from build123d import *

# Parameters (mm, degrees)
SKETCH_1_R          = 17.5
EXTRUDE_1_DEPTH     = 3.65
SKETCH_3_R          = 1.25
CUT_EXTRUDE_1_DEPTH = 5
CHAMFER_1_SIZE      = 0.5
SKETCH_4_R          = 1.5
CUT_EXTRUDE_2_DEPTH = 10
SKETCH_5_R          = 2.75
CUT_EXTRUDE_3_DEPTH = 10


with BuildPart() as part:
    # 草图1 → 凸台-拉伸1 (new body)
    with BuildSketch(Plane.XY):
        Circle(SKETCH_1_R)
    extrude(amount=EXTRUDE_1_DEPTH)

    # 草图3 → 切除-拉伸1 (cut)
    with BuildSketch(Plane(origin=(0, 0, 0), x_dir=(-1, 0, 0), z_dir=(0, 0, -1))):
        with Locations((0, 13.5)):
            Circle(SKETCH_3_R)
        with Locations((9.545941546, 9.545941546)):
            Circle(SKETCH_3_R)
        with Locations((13.5, 0)):
            Circle(SKETCH_3_R)
        with Locations((9.545941546, -9.545941546)):
            Circle(SKETCH_3_R)
        with Locations((0, -13.5)):
            Circle(SKETCH_3_R)
        with Locations((-9.545941546, -9.545941546)):
            Circle(SKETCH_3_R)
        with Locations((-13.5, 0)):
            Circle(SKETCH_3_R)
        with Locations((-9.545941546, 9.545941546)):
            Circle(SKETCH_3_R)
    extrude(amount=-CUT_EXTRUDE_1_DEPTH, mode=Mode.SUBTRACT)

    # 倒角1
    chamfer_1_edges = [part.edges().sort_by_distance(p)[0] for p in [
        (-17.5, 0, 0),
        (-17.5, 0, 3.65),
    ]]
    chamfer(chamfer_1_edges, length=CHAMFER_1_SIZE)

    # 草图4 → 切除-拉伸2 (cut)
    with BuildSketch(Plane(origin=(0, 0, 0), x_dir=(-1, 0, 0), z_dir=(0, 0, -1))):
        with Locations((0, 7)):
            Circle(SKETCH_4_R)
        with Locations((7, 0)):
            Circle(SKETCH_4_R)
        with Locations((0, -7)):
            Circle(SKETCH_4_R)
        with Locations((-7, 0)):
            Circle(SKETCH_4_R)
    extrude(amount=-CUT_EXTRUDE_2_DEPTH, mode=Mode.SUBTRACT)

    # 草图5 → 切除-拉伸3 (cut)
    with BuildSketch(Plane(origin=(0, 0, 0), x_dir=(-1, 0, 0), z_dir=(0, 0, -1))):
        Circle(SKETCH_5_R)
    extrude(amount=-CUT_EXTRUDE_3_DEPTH, mode=Mode.SUBTRACT)


solid = part.part
Read the model definition and answer for the solid it produces. Units are mm, in the model's axes. Coordinates: 2 decimals unless noted, no trailing zeros. Loops run counter-clockwise (first coordinate to the right, second up) from the corner with the lowest first, then second, coordinate; pieces in that order, holes last. Notation, with made-up numbers: (31, 29.25) -> (41, 29.25) arc R20 ccw to (41, 58.25) -> close; hole circle Ø11 at (21.5, 52.25). An arc over 180 degrees is marked (long way). Write item = value, one per line. Start each with the question number.
1) The part is cut by section A-A, the plane y = 0. Determine the outline of the cut face in (x, z), plus the area to 3 significant figures.
2) Find the intervals of material crossed by L1, parallel to X at y = 10, z = 1.9; L2, parallel to Y at x = 9, z = 0.55; L3, parallel to Y at x = 9.5, z = 1.95, in increasing order. Write a range as from..to.
3) Given P1, Ø2, axis at x = 0, y = 13.5, coming from the -Z side; P2, Ø1, axis at y = -12.5, z = 3, coming from the +X side, each flat-ended and moving along its own axis, determine where each tip first touches the part or whether it passes through.
4) The mould has two halves that part along Y. Classify faces 1 (the face through (-13.887, -10.648, 1.806)), 2 (the face through (0.16, -12.26, 1.8)), 3 (the face through (-12.25, 0.05, 1.8)), 4 (the face through (4, 0, 0)): pulls with the +Y half, pulls with the -Y half, needs draft (parallel to the pull), parting line crosses it, or undercut.
5) The part is cut by section B-B, the plane z = 2.7. State how many separate pieces and enclosed holes the cut face has, plus the area to 3 significant figures.
Result:
q1.outline = (-17.5, 0.5) -> (-17, 0) -> (-14.75, 0) -> (-14.75, 3.65) -> (-17, 3.65) -> (-17.5, 3.15) -> close; (-12.25, 0) -> (-8.5, 0) -> (-8.5, 3.65) -> (-12.25, 3.65) -> close; (-5.5, 0) -> (-2.75, 0) -> (-2.75, 3.65) -> (-5.5, 3.65) -> close; (2.75, 0) -> (5.5, 0) -> (5.5, 3.65) -> (2.75, 3.65) -> close; (8.5, 0) -> (12.25, 0) -> (12.25, 3.65) -> (8.5, 3.65) -> close; (14.75, 0) -> (17, 0) -> (17.5, 0.5) -> (17.5, 3.15) -> (17, 3.65) -> (14.75, 3.65) -> close
q1.area = 67.0 mm²
q2.L1 = -14.36..-10.71, -8.38..8.38, 10.71..14.36
q2.L2 = -15.01..-10.67, -8.42..8.42, 10.67..15.01
q2.L3 = -14.7..-10.8, -8.3..8.3, 10.8..14.7
q3.P1 = through
q3.P2 = 12.74
q4.face_1 = parting line crosses it
q4.face_2 = undercut
q4.face_3 = undercut
q4.face_4 = needs draft
q5.separate_pieces = 1
q5.enclosed_holes = 13
q5.area = 871 mm²
